The drawing under review shows one solid part. Ordinate dimensions are in mm from its lowest x, y, z. A direction names the side the tool comes from. Round coordinates to 2 decimals unless told otherwise and drop trailing zeros. Write each loop counter-clockwise with the first axis right and the second up, starting at its lowest first coordinate (ties: lowest second). Pieces come first, ordered by that corner, then holes. Notation, with made-up numbers: (-39, -11.5) - (-33, -11.5) arc R35 ccw to (-33, 22.5) - close; hole circle Ø4 at (8, 74). An arc over 180 degrees is marked (long way). One line per question, with ' | ' between items. Start each with the question number.
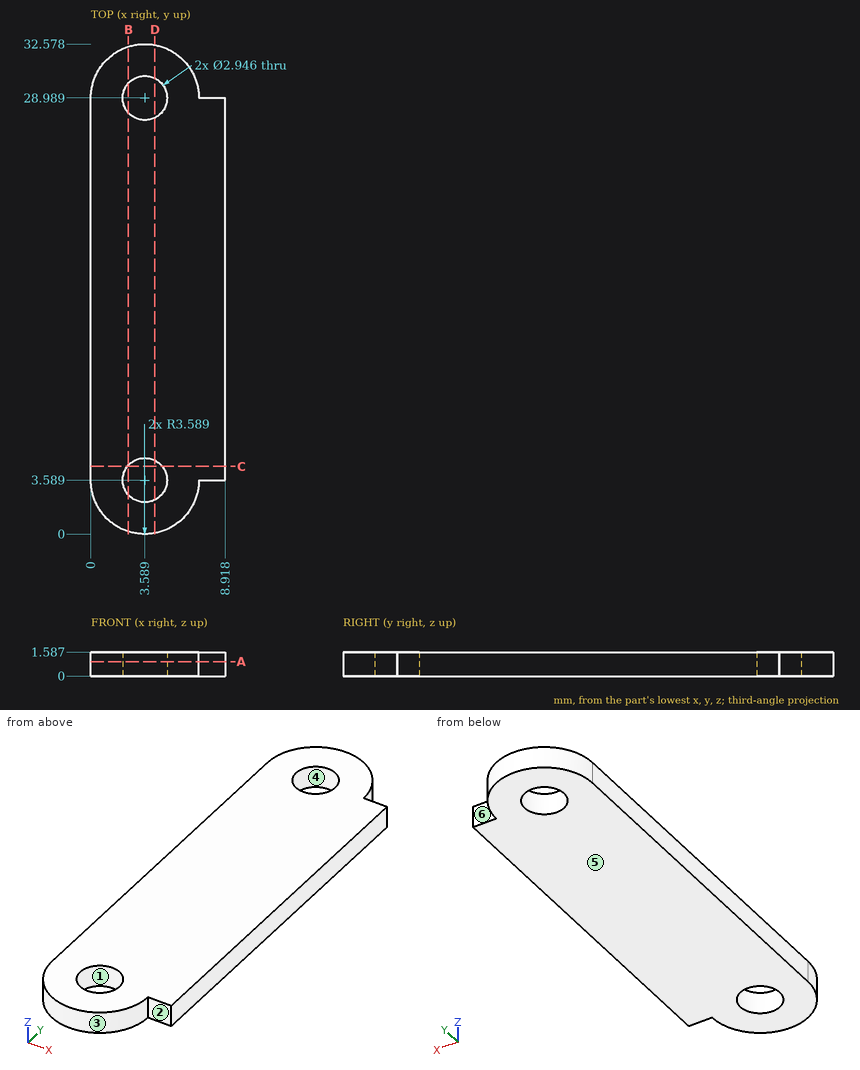
1. Add section A-A, the plane z = 0.95. Write out the cut boundary in (x, y) (1 decimal).
2. The part is to be moulded in two halves that separate along Y. For the marked faces 3, 4, 5 and 6, say which applies: pulls with the +Y half, pulls with the -Y half, needs draft (parallel to the pull), parting line crosses it, or undercut.
3. Clearance check with flat-ended pins moving along their axes: P1, Ø0.5, axis at x = 8, z = 1, coming from the +Y side; P2, Ø0.8, axis at x = 8, z = 1, coming from the -Y side. State where each tip first meets the part, or that it passes through.
4. Wall thickness on line 1 along Y through (x, z) = (4.5, 1) (1 decimal); line 2 along Y through (x, z) = (3.25, 0.1) (1 decimal); line 3 along X through (y, z) = (3, 1.1): over which ranges is each line inside the solid? List them lowest first. Write a range as [from, to].
5. Add section D-D, the plane x = 4.25. Write out the cut boundary in (y, z) (1 decimal).
6. Machinability: for the marked faces 1 and 2, which of the approach directions +Z, -Z, +X, -X, +Y, -Y give a long, thin tool a straight path to every point of the face, cutting with its end or side? Answer none if there is none.
7. Add section B-B, the plane x = 2.5. Write out the cut boundary in (y, z).
8. Add section C-C, the plane y = 4.5. Write out the cut boundary in (x, z), then the cut area to 3 significant figures.
Geometry check:
1) outline: (0, 3.6) arc R3.6 ccw to (7.2, 3.6) - (8.9, 3.6) - (8.9, 29) - (7.2, 29) arc R3.6 ccw to (0, 29) - close; hole circle Ø2.9 at (3.6, 3.6); hole circle Ø2.9 at (3.6, 29)
2) face 3: pulls with the -Y half | face 4: undercut | face 5: needs draft | face 6: pulls with the +Y half
3) P1: stops at y = 28.99 | P2: stops at y = 3.59
4) line 1: y = [0.1, 2.4], [4.7, 27.8], [30.1, 32.5] | line 2: y = [0, 2.2], [5, 27.6], [30.4, 32.6] | line 3: x = [0.05, 2.24], [4.94, 7.13]
5) outline: (0.1, 0) - (2.3, 0) - (2.3, 1.6) - (0.1, 1.6) - close; (4.9, 0) - (27.7, 0) - (27.7, 1.6) - (4.9, 1.6) - close; (30.3, 0) - (32.5, 0) - (32.5, 1.6) - (30.3, 1.6) - close
6) face 1: +Z, -Z | face 2: +Z, -Z, +X, -Y
7) outline: (0.17, 0) - (2.6, 0) - (2.6, 1.59) - (0.17, 1.59) - close; (4.58, 0) - (28, 0) - (28, 1.59) - (4.58, 1.59) - close; (29.98, 0) - (32.41, 0) - (32.41, 1.59) - (29.98, 1.59) - close
8) outline: (0, 0) - (2.43, 0) - (2.43, 1.59) - (0, 1.59) - close; (4.75, 0) - (8.92, 0) - (8.92, 1.59) - (4.75, 1.59) - close | area: 10.5 mm2
